Could you check a few things on this drawing? It's one solid part, dimensions in mm from its lowest x, y, z. Give positions to 0.01 mm unless a question says otherwise; leave off trailing zeros. Order: outer loops, then holes, each group sorted by start corner. A loop starts at its lowest first (then second) coordinate and runs counter-clockwise, first axis right, second up.
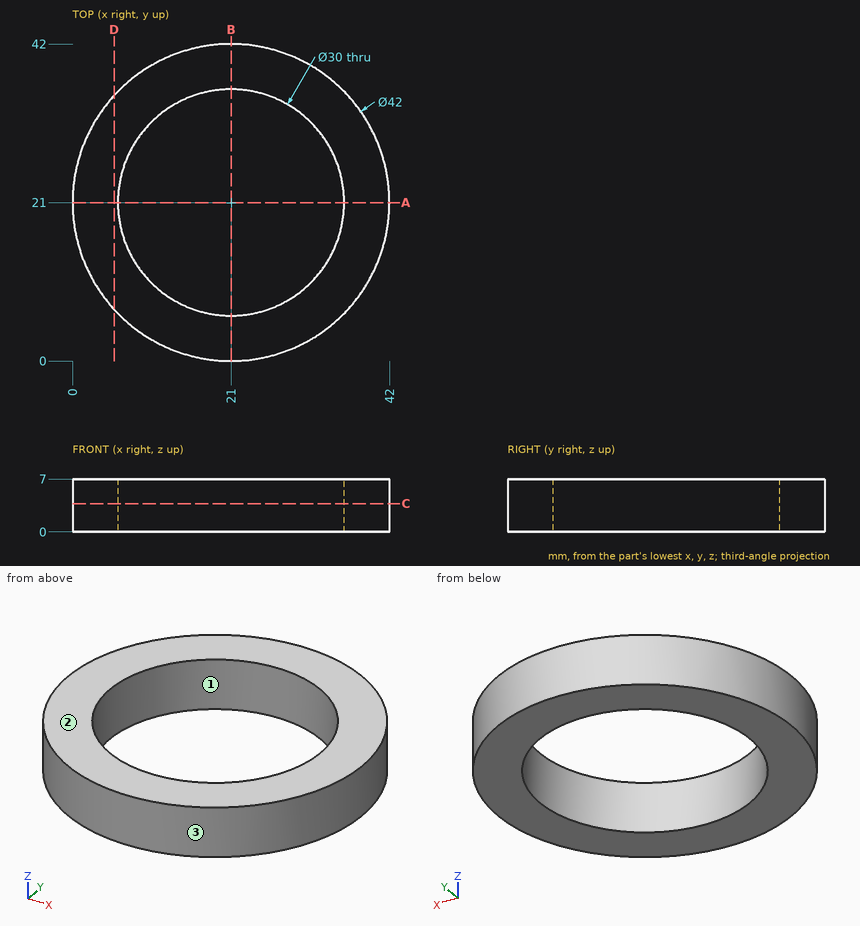
Q1. I'm going to push flat-ended pins straight in: P1, Ø4, axis at x = 6, z = 2.5, coming from the +Y side; P2, Ø3, axis at x = 36, z = 1, coming from the -Y side; P3, Ø2, axis at x = 36, z = 4.5, coming from the -Y side; P4, Ø3, axis at x = 34, y = 23, coming from the +Z side. Where does each tip first touch, or does it pass through?
Filled sheet:
P1: stops at y = 37.49
P2: stops at y = 4.91
P3: stops at y = 5.35
P4: passes through
Q2. I need wall thicknesses on L1, parallel to Y at x = 21, z = 1.5; L2, parallel to Y at x = 30, z = 6.75; L3, parallel to X at y = 23, z = 1.75. Which ranges of each line are inside material? Lowest first, please.
Filled sheet:
L1: y = 0 to 6, 36 to 42
L2: y = 2.03 to 9, 33 to 39.97
L3: x = 0.1 to 6.13, 35.87 to 41.9
Q3. Thinking about a two-plate mould opening in X: for the marked faces 1, 2 and 3, which applies, released by +X, released by -X, zero draft, split by the parting line, or undercut?
Filled sheet:
face 1: undercut
face 2: zero draft
face 3: split by the parting line
Q4. If we section it at A-A on y = 21: List the corners of the cut face in (x, z) for me, plus the area to 3 significant figures.
Filled sheet:
outline: (0, 0) - (6, 0) - (6, 7) - (0, 7) - close; (36, 0) - (42, 0) - (42, 7) - (36, 7) - close
area: 84.0 mm2
Q5. If we section it at D-D on x = 5.5: List the corners of the cut face in (y, z) for me, plus the area to 3 significant figures.
Filled sheet:
outline: (6.83, 0) - (35.17, 0) - (35.17, 7) - (6.83, 7) - close
area: 198 mm2
Q6. If we section it at C-C on z = 3.75: List the corners of the cut face in (x, y) for me.
Filled sheet:
outline: circle Ø42 at (21, 21); hole circle Ø30 at (21, 21)
